```python
from build123d import *

# Parameters (mm, degrees)
SKETCH1_W           = 48
SKETCH1_H           = 12
BOSS_EXTRUDE1_DEPTH = 36
SKETCH1_3_W         = 48
SKETCH1_3_H         = 12
BOSS_EXTRUDE2_DEPTH = 12
BOSS_EXTRUDE4_START = -12
SKETCH1_5_W         = 48
SKETCH1_5_H         = 16
BOSS_EXTRUDE4_DEPTH = 24


with BuildPart() as part:
    # Sketch1 → Boss-Extrude1 (new body)
    with BuildSketch(Plane.XY):
        with Locations((24, 18)):
            Rectangle(SKETCH1_W, SKETCH1_H)
        Polygon((0, 12), (0, 0), (72, 0), (72, 24), (48, 24), (48, 12), align=None)
    extrude(amount=-BOSS_EXTRUDE1_DEPTH)

    # Sketch1_3 → Boss-Extrude2 (add)
    with BuildSketch(Plane.XY):
        with Locations((24, 18)):
            Rectangle(SKETCH1_3_W, SKETCH1_3_H)
    extrude(amount=BOSS_EXTRUDE2_DEPTH)

    # Sketch1_5 → Boss-Extrude4 (add)
    with BuildSketch(Plane.XY.offset(BOSS_EXTRUDE4_START)):
        with Locations((24, 32)):
            Rectangle(SKETCH1_5_W, SKETCH1_5_H)
    extrude(amount=-BOSS_EXTRUDE4_DEPTH)


solid = part.part
```
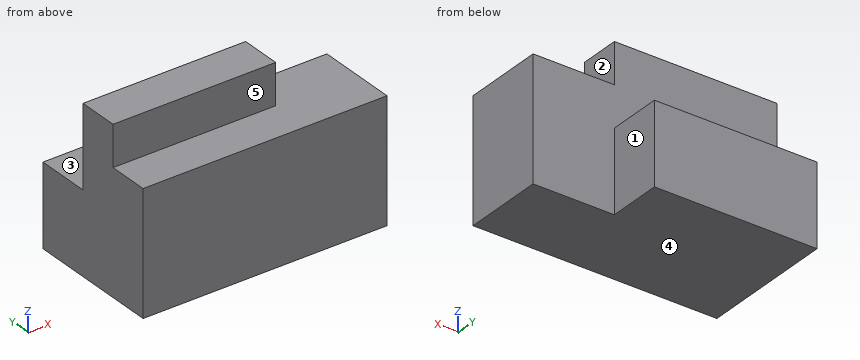
The listing builds one solid part. Answer for the finished solid, in the listing's coordinates (mm). Face numbers are marked on the shaded views. A direction names the side the tool comes from. Round coordinates to 2 decimals unless told otherwise and drop trailing zeros. Loops run counter-clockwise (first coordinate to the right, second up) from the corner with the lowest first, then second, coordinate; pieces in that order, holes last.
1) A cutting plane is placed at A-A on x = 10.5. Determine the outline of the cut face in (y, z).
Outcome:
outline: (0, -36) - (40, -36) - (40, -12) - (24, -12) - (24, 12) - (12, 12) - (12, 0) - (0, 0) - close
2) A cutting plane is placed at B-B on z = 1. Determine the outline of the cut face in (x, y), plus the area to 3 significant figures.
Outcome:
outline: (0, 12) - (48, 12) - (48, 24) - (0, 24) - close
area: 576 mm2
3) A cutting plane is placed at D-D on z = -24. Determine the outline of the cut face in (x, y), plus the area to 3 significant figures.
Outcome:
outline: (0, 0) - (72, 0) - (72, 24) - (48, 24) - (48, 40) - (0, 40) - close
area: 2,500 mm2
4) Consider line 1 (X direction, y = 38, z = -17); line 2 (Z direction, x = 45, y = 30); line 3 (Z direction, x = 67, y = 16.5). Determine where each line is inside the solid, lowest interval first.
Outcome:
line 1: x = 0 to 48
line 2: z = -36 to -12
line 3: z = -36 to 0
5) Given P1, Ø17.5, axis at y = 35, z = -27.5, coming from the +X side; P2, Ø2, axis at x = 18, z = -1.5, coming from the +Y side; P3, Ø6, axis at x = 40.5, y = 33, coming from the +Z side, each flat-ended and moving along its own axis, determine where each tip first touches the part or whether it passes through.
Outcome:
P1: stops at x = 48
P2: stops at y = 24
P3: stops at z = -12
6) A cutting plane is placed at C-C on y = 27. Determine the outline of the cut face in (x, z), plus the area to 3 significant figures.
Outcome:
outline: (0, -36) - (48, -36) - (48, -12) - (0, -12) - close
area: 1,150 mm2
7) For the marked faces 1, 2, 3, 4 and 5, determine the directions among +Z, -Z, +X, -X, +Y, -Y from which every point of the face is accessible in a straight line to the end or side of a thin tool.
Outcome:
face 1: +Z, -Z, +X, +Y
face 2: +Z, +X, +Y, -Y
face 3: +Z, +X, -X, +Y
face 4: -Z, +X, -X, +Y, -Y
face 5: +Z, +X, -X, -Y
